Geometry: final body of the model. Coordinates: model frame, mm. Coordinates: 2 decimals unless noted, no trailing zeros. Order: outer loops, then holes, each group sorted by start corner. A loop starts at its lowest first (then second) coordinate and runs counter-clockwise, first axis right, second up. Notation, with made-up numbers: (7.5, -0.75) -> (22.5, -0.75) arc R11 cw to (22.5, 6.25) -> close; hole circle Ø10 at (12, 48). An arc over 180 degrees is marked (long way). Use one line per item in the form item = value.
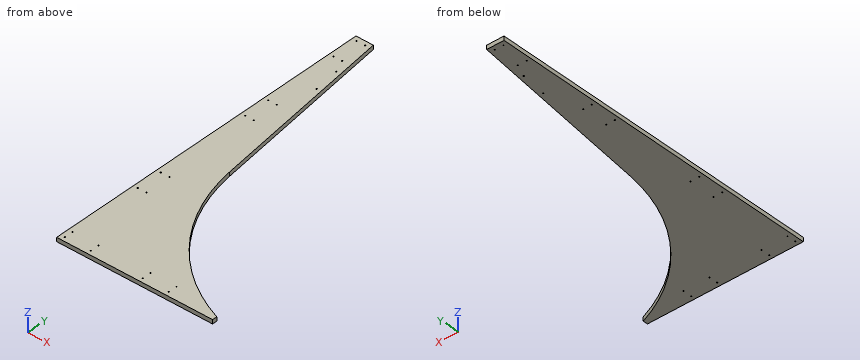
```python
from build123d import *

# Parameters (mm, degrees)
BOSS_EXTRUDE1_DEPTH = 11.90625
SKETCH2_R           = 1.5875
CUT_EXTRUDE1_DEPTH  = 12.90625
SKETCH3_R           = 1.5875
CUT_EXTRUDE2_DEPTH  = 12.90625


with BuildPart() as part:
    # Sketch1 → Boss-Extrude1 (new body)
    with BuildSketch(Plane.XY):
        with BuildLine():
            Line((0, 990.6), (0, 0))
            Line((0, 0), (457.201, 0))
            Line((457.201, 0), (457.201, 13.862038208))
            ThreePointArc((457.201, 13.862038208), (232.767577124, 176.628269142), (124.367415652, 431.8))
            Line((124.367415652, 431.8), (50.8, 990.6))
            Line((50.8, 990.6), (0, 990.6))
        make_face()
    extrude(amount=BOSS_EXTRUDE1_DEPTH)

    # Sketch2 → Cut-Extrude1 (cut, through all)
    with BuildSketch(Plane.XY.offset(11.90625)):
        with Locations((12.7, 977.9)):
            Circle(SKETCH2_R)
        with Locations((38.1, 977.9)):
            Circle(SKETCH2_R)
        with Locations((12.7, 901.7)):
            Circle(SKETCH2_R)
        with Locations((38.1, 901.7)):
            Circle(SKETCH2_R)
        with Locations((12.7, 609.6)):
            Circle(SKETCH2_R)
        with Locations((38.1, 609.6)):
            Circle(SKETCH2_R)
        with Locations((12.7, 685.8)):
            Circle(SKETCH2_R)
        with Locations((38.1, 685.8)):
            Circle(SKETCH2_R)
        with Locations((12.7, 254)):
            Circle(SKETCH2_R)
        with Locations((38.1, 254)):
            Circle(SKETCH2_R)
        with Locations((12.7, 330.2)):
            Circle(SKETCH2_R)
        with Locations((38.1, 330.2)):
            Circle(SKETCH2_R)
        with Locations((12.7, 38.1)):
            Circle(SKETCH2_R)
        with Locations((12.7, 12.7)):
            Circle(SKETCH2_R)
        with Locations((88.9, 38.1)):
            Circle(SKETCH2_R)
        with Locations((88.9, 12.7)):
            Circle(SKETCH2_R)
        with Locations((241.3, 38.1)):
            Circle(SKETCH2_R)
        with Locations((317.5, 38.1)):
            Circle(SKETCH2_R)
        with Locations((241.3, 12.7)):
            Circle(SKETCH2_R)
        with Locations((317.5, 12.7)):
            Circle(SKETCH2_R)
    extrude(amount=-CUT_EXTRUDE1_DEPTH, mode=Mode.SUBTRACT)

    # Sketch3 → Cut-Extrude2 (cut, through all)
    with BuildSketch(Plane.XY.offset(11.90625)):
        with Locations((64.74219971, 787.4)):
            Circle(SKETCH3_R)
        with Locations((54.710279394, 863.6)):
            Circle(SKETCH3_R)
    extrude(amount=-CUT_EXTRUDE2_DEPTH, mode=Mode.SUBTRACT)


solid = part.part
```
1) Contact query for a flat-ended pin moving along its axis: P1, Ø1, axis at y = 545, z = 4.5, coming from the +X side. Output: stop coordinate, or through.
Results found:
P1 = 109.53
2) Section C-C, the plane x = 148. Output: boundary loops of the cut face in (y, z), and give its area (3 significant figures).
Results found:
outline = (0, 0) -> (331.21, 0) -> (331.21, 11.91) -> (0, 11.91) -> close
area = 3,940 mm2
3) Section B-B, the plane y = 637. Output: boundary loops of the cut face in (x, z), and give its area (3 significant figures).
Results found:
outline = (0, 0) -> (97.35, 0) -> (97.35, 11.91) -> (0, 11.91) -> close
area = 1,160 mm2
4) Section A-A, the plane z = 5.5. Give the number of separate pieces and of enclosed holes in the cut face, and give its area (3 significant figures).
Results found:
separate_pieces = 1
enclosed_holes = 22
area = 150,000 mm2
5) Material intervals for probe 1 along Y at (x, z) = (399, 4.25); probe 2 along Y at (x, z) = (241.3, 4.25); probe 3 along X at (y, z) = (330.2, 7.5), sorted ascending. Write a range as from..to.
Results found:
probe_1 = 0..39.72
probe_2 = 0..11.11, 14.29..36.51, 39.69..166.2
probe_3 = 0..11.11, 14.29..36.51, 39.69..148.35
